Geometry check sheet. Reference: the model listing, model coordinates, mm. Give positions to 0.01 mm unless a question says otherwise; leave off trailing zeros. Order: outer loops, then holes, each group sorted by start corner. A loop starts at its lowest first (then second) coordinate and runs counter-clockwise, first axis right, second up. Notation, with made-up numbers: M 23.25,33.5 L 70.25,33.5 A12 ccw 70.25,50.5 Z; hole C 64.5,82 d5. An arc over 180 degrees is marked long. Answer as a JSON object with one key per item and string values. Group by question number.
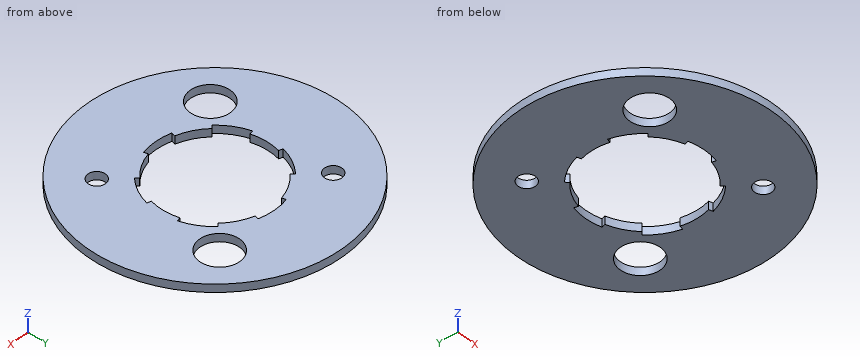
from build123d import *

# Parameters (mm, degrees)
F0_R     = 25.3907018743
F0_R_2   = 3.96875
F0_R_3   = 1.7272
F0_R_4   = 11.1125
F1_DEPTH = 1.5875
F3_DEPTH = 1.5875
F4_COUNT = 6
F4_ANGLE = 300


with BuildPart() as f1:
    # F0 (on Top) → F1 (new body)
    with BuildSketch(Plane.XY):
        Circle(F0_R)
        with Locations((-12.3478521665, -12.3478521665)):
            Circle(F0_R_2, mode=Mode.SUBTRACT)
        with Locations((12.3478521665, -12.3478521665)):
            Circle(F0_R_3, mode=Mode.SUBTRACT)
        with Locations((-12.3478521665, 12.3478521665)):
            Circle(F0_R_3, mode=Mode.SUBTRACT)
        Circle(F0_R_4, mode=Mode.SUBTRACT)
        with Locations((12.3478521665, 12.3478521665)):
            Circle(F0_R_2, mode=Mode.SUBTRACT)
    extrude(amount=F1_DEPTH)

    # F2 (on face) → F3 (cut, through all)
    with BuildSketch(Plane.XY.offset(1.5875)):
        with BuildLine():
            ThreePointArc((-2.8761266387, 10.7338507446), (0, 11.1125), (2.8761266387, 10.7338507446))
            Line((2.8761266387, 10.7338507446), (3.0815642558, 11.5005543693))
            ThreePointArc((3.0815642558, 11.5005543693), (0, 11.90625), (-3.0815642558, 11.5005543693))
            Line((-3.0815642558, 11.5005543693), (-2.8761266387, 10.7338507446))
        make_face()
    f3 = extrude(amount=-F3_DEPTH, mode=Mode.SUBTRACT)

    # F4: F3 ×6 about axis
    f4_axis = Axis((0, 0, 0), (0, 0, -1))
    for i in range(1, F4_COUNT):
        add(f3.rotate(f4_axis, i * F4_ANGLE / (F4_COUNT - 1)), mode=Mode.SUBTRACT)


solid = f1.part
1. Thickness scan on line 1 along Y through (x, z) = (-12, 0.8); line 2 along Y through (x, z) = (0.5, 0.25); line 3 along X through (y, z) = (9.5, 0.35). Record the ranges inside material, lowest first. Write a range as [from, to].
2. Cross-section at D-D (z = 0.4). State how many separate pieces and enclosed holes the cut face has, and give its area (3 significant figures).
3. Cross-section at A-A (x = 0). Record the cut outline in (y, z), and give its area (3 significant figures).
4. Cross-section at C-C (y = 9.5). Record the cut outline in (x, z), and give its area (3 significant figures).
5. Depth check by flat-ended pin: pin 1 (3 mm diameter, centred on x = 12.35, y = -12.35, fed in from +Z); pin 2 (12.5 mm diameter, centred on x = -12.35, y = -12.35, fed in from -Z). Enter the tip coordinate at first touch or a pass-through.
6. Cross-section at B-B (y = 0). Record the cut outline in (x, z).
Report:
{
 "1": {"line 1": "y = [-22.38, -16.3], [-8.39, 10.66], [14.04, 22.38]", "line 2": "y = [-25.39, -11.9], [11.9, 25.39]", "line 3": "x = [-23.55, -5.77], [5.77, 9.58], [15.11, 23.55]"},
 "2": {"separate pieces": "1", "enclosed holes": "5", "area": "1,490 mm2"},
 "3": {"outline": "M -25.39,0 L -11.91,0 L -11.91,1.59 L -25.39,1.59 Z; M 11.91,0 L 25.39,0 L 25.39,1.59 L 11.91,1.59 Z", "area": "42.8 mm2"},
 "4": {"outline": "M -23.55,0 L -5.77,0 L -5.77,1.59 L -23.55,1.59 Z; M 5.77,0 L 9.58,0 L 9.58,1.59 L 5.77,1.59 Z; M 15.11,0 L 23.55,0 L 23.55,1.59 L 15.11,1.59 Z", "area": "47.7 mm2"},
 "5": {"pin 1": "passes through", "pin 2": "stops at z = 0"},
 "6": {"outline": "M -25.39,0 L -11.11,0 L -11.11,1.59 L -25.39,1.59 Z; M 11.11,0 L 25.39,0 L 25.39,1.59 L 11.11,1.59 Z"}
}
